Design review of the part built by this model. Coordinates are the model's own, in mm. Face numbers are marked on the shaded views. Coordinates: 2 decimals unless noted, no trailing zeros. Order: outer loops, then holes, each group sorted by start corner. A loop starts at its lowest first (then second) coordinate and runs counter-clockwise, first axis right, second up. Notation, with made-up numbers: M 41.5,-17 L 54.5,-17 A30 ccw 54.5,21 Z; hole C 9,-8.5 d4. An arc over 180 degrees is marked long. Answer as a JSON object with one key per item and string values.
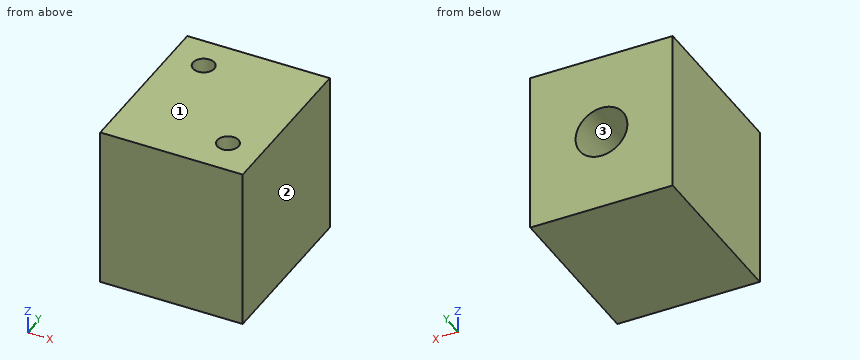
from build123d import *

# Parameters (mm, degrees)
SKETCH1_W           = 22
SKETCH1_H           = 25
BOSS_EXTRUDE1_DEPTH = 26
SKETCH2_R           = 4
CUT_EXTRUDE2_DEPTH  = 17
SKETCH3_R           = 1.65
CUT_EXTRUDE3_DEPTH  = 10


with BuildPart() as part:
    # Sketch1 → Boss-Extrude1 (new body)
    with BuildSketch(Plane(origin=(0, 0, 0), x_dir=(1, 0, 0), z_dir=(0, 1, 0))):
        Rectangle(SKETCH1_W, SKETCH1_H)
    extrude(amount=BOSS_EXTRUDE1_DEPTH)

    # Sketch2 → Cut-Extrude2 (cut)
    with BuildSketch(Plane(origin=(0, 26, 0), x_dir=(1, 0, 0), z_dir=(0, 1, 0))):
        with Locations(Location((0, 0, 0), (0, 0, 270))):
            Circle(SKETCH2_R)
    extrude(amount=-CUT_EXTRUDE2_DEPTH, mode=Mode.SUBTRACT)

    # Sketch3 → Cut-Extrude3 (cut)
    with BuildSketch(Plane.XY.offset(12.5)):
        with Locations((-5.75, 20.75)):
            Circle(SKETCH3_R)
        with Locations((5.75, 5.75)):
            Circle(SKETCH3_R)
    extrude(amount=-CUT_EXTRUDE3_DEPTH, mode=Mode.SUBTRACT)


solid = part.part
1) Mouldability with a two-part tool opening along X and no side actions: class the marked faces 1, 2 and 3 as released by +X, released by -X, zero draft, split by the parting line, or undercut.
Taken from the geometry:
{"face 1": "zero draft", "face 2": "released by +X", "face 3": "undercut"}
2) Insertion check: pin 1 Ø2.5 at (x, y) = (-6, 20) entering from +Z; pin 2 Ø2.5 at (x, z) = (0.5, -1.5) entering from +Y. Each pin has a flat end and moves straight along its axis. Give the tip position at first contact, or say it passes through.
Taken from the geometry:
{"pin 1": "stops at z = 12.5", "pin 2": "stops at y = 9"}
3) Add section C-C (x = 0). State the section outline as (y, z) points, and give its area (3 significant figures).
Taken from the geometry:
{"outline": "M 0,-12.5 L 26,-12.5 L 26,-4 L 9,-4 L 9,4 L 26,4 L 26,12.5 L 0,12.5 Z", "area": "514 mm2"}
4) Add section A-A (y = 15.75). State the section outline as (x, z) points.
Taken from the geometry:
{"outline": "M -11,-12.5 L 11,-12.5 L 11,12.5 L -11,12.5 Z; hole C 0,0 d8"}
5) Add section D-D (z = 3). State the section outline as (x, y) points, and give its area (3 significant figures).
Taken from the geometry:
{"outline": "M -11,0 L 11,0 L 11,26 L 2.65,26 L 2.65,9 L -2.65,9 L -2.65,26 L -11,26 Z; hole C -5.75,20.75 d3.3; hole C 5.75,5.75 d3.3", "area": "465 mm2"}
6) Add section B-B (z = 0). State the section outline as (x, y) points, and give its area (3 significant figures).
Taken from the geometry:
{"outline": "M -11,0 L 11,0 L 11,26 L 4,26 L 4,9 L -4,9 L -4,26 L -11,26 Z", "area": "436 mm2"}
7) To check wall thickness, follow L1, parallel to Y at x = -5.75, z = 8; L2, parallel to X at y = 19.75, z = 0; L3, parallel to Y at x = 5, z = 10. State the ranges of each line that lie inside material, in increasing order.
Taken from the geometry:
{"L1": "y = 0 to 19.1, 22.4 to 26", "L2": "x = -11 to -4, 4 to 11", "L3": "y = 0 to 4.28, 7.22 to 26"}
